CAD build for the part. Positions are in the model's coordinates, mm. Face numbers are marked on the shaded views. Coordinates: 2 decimals unless noted, no trailing zeros. Write each loop counter-clockwise with the first axis right and the second up, starting at its lowest first coordinate (ties: lowest second). Pieces come first, ordered by that corner, then holes. Notation, with made-up numbers: (-17, 31.25) - (-6, 31.25) arc R19 cw to (-6, 54.25) - close; hole circle Ø8 at (65.25, -24.5). An arc over 180 degrees is marked (long way). One line per question, with ' | ' between items. Start each with the question number.
1. Probe line 1 (X direction, y = 1.5, z = 3.75) (3 decimals); line 2 (Y direction, x = 0, z = 4.75); line 3 (X direction, y = -5, z = 2.75) (3 decimals). List the from-to ranges inside material, lowest first.
2. Band-saw the part on B-B, the plane x = 0. Write the cut outline in (y, z).
3. Two-plate mould, pull along X, no slides. Class the marked faces 1, 2, 3 and 4: +X half, -X half, draft (parallel to the pull), parting line (faces both ways), or undercut.
4. Flat gauge pin, fed straight in: P1, Ø8.5, axis at x = 15.525, y = 0, coming from the -Z side. Where does the tip first touch, or does it go through?
5. Band-saw the part on A-A, the plane y = 0. Give the number of separate pieces and of enclosed holes in the cut face, then the cut area to 3 significant figures.
from build123d import *

# Parameters (mm, degrees)
SKETCH1_W                 = 48.505
SKETCH1_H                 = 19.05
BOSS_EXTRUDE1_DEPTH       = 6.35
F_6_CLEARANCE_HOLE1_D     = 3.6576
F_6_CLEARANCE_HOLE1_DEPTH = 9.398
F_6_CLEARANCE_HOLE1_TIP   = 1.0988539
SKETCH4_R                 = 4.7625
CUT_EXTRUDE1_DEPTH        = 2
F_6_32_TAPPED_HOLE1_D     = 2.7051
F_6_32_TAPPED_HOLE1_DEPTH = 10.9728
F_6_32_TAPPED_HOLE1_TIP   = 0.81269403


with BuildPart() as part:
    # Sketch1 → Boss-Extrude1 (new body)
    with BuildSketch(Plane.XY):
        with Locations((3.2525, -3.175)):
            Rectangle(SKETCH1_W, SKETCH1_H)
    extrude(amount=BOSS_EXTRUDE1_DEPTH)

    # #6 Clearance Hole1
    with Locations(Plane.XY.offset(6.35)):
        with Locations((-15.525, 0), (15.525, 0)):
            Hole(F_6_CLEARANCE_HOLE1_D / 2, depth=F_6_CLEARANCE_HOLE1_DEPTH)
            with Locations((0, 0, -(F_6_CLEARANCE_HOLE1_DEPTH + F_6_CLEARANCE_HOLE1_TIP / 2))):  # 118° drill point
                Cone(0, F_6_CLEARANCE_HOLE1_D / 2, F_6_CLEARANCE_HOLE1_TIP, mode=Mode.SUBTRACT)

    # Sketch4 → Cut-Extrude1 (cut)
    with BuildSketch(Plane(origin=(0, 0, 0), x_dir=(-1, 0, 0), z_dir=(0, 0, -1))):
        with Locations((-15.525, 0)):
            Circle(SKETCH4_R)
        with Locations((15.525, 0)):
            Circle(SKETCH4_R)
    extrude(amount=-CUT_EXTRUDE1_DEPTH, mode=Mode.SUBTRACT)

    # #6-32 Tapped Hole1
    with Locations(Plane(origin=(0, 0, 0), x_dir=(-1, 0, 0), z_dir=(0, 0, -1))):
        with Locations((0, -4.8294)):
            Hole(F_6_32_TAPPED_HOLE1_D / 2, depth=F_6_32_TAPPED_HOLE1_DEPTH)
            with Locations((0, 0, -(F_6_32_TAPPED_HOLE1_DEPTH + F_6_32_TAPPED_HOLE1_TIP / 2))):  # 118° drill point
                Cone(0, F_6_32_TAPPED_HOLE1_D / 2, F_6_32_TAPPED_HOLE1_TIP, mode=Mode.SUBTRACT)


solid = part.part
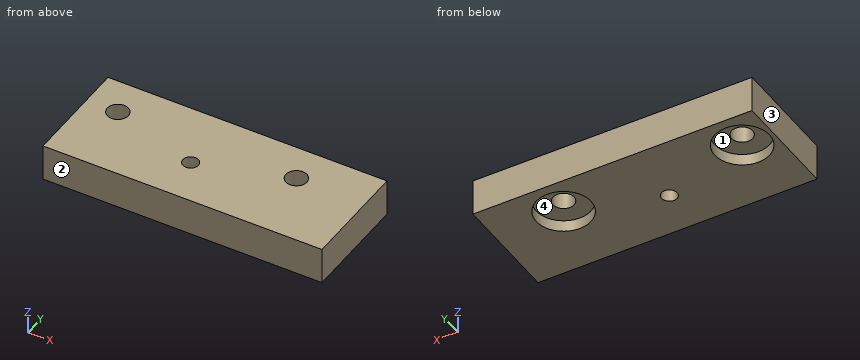
Filled in:
1) line 1: x = -21 to -16.571, -14.479 to 14.479, 16.571 to 27.505 | line 2: y = -12.7 to -6.18, -3.48 to 6.35 | line 3: x = -21 to -1.342, 1.342 to 27.505
2) outline: (-12.7, 0) - (-6.18, 0) - (-6.18, 6.35) - (-12.7, 6.35) - close; (-3.48, 0) - (6.35, 0) - (6.35, 6.35) - (-3.48, 6.35) - close
3) face 1: undercut | face 2: draft | face 3: -X half | face 4: undercut
4) P1: stops at z = 2
5) separate pieces: 3 | enclosed holes: 0 | area: 238 mm²
